from build123d import *

# Parameters (mm, degrees)
CROQUIS1_W              = 30
CROQUIS1_H              = 20
SALIENTE_EXTRUIR1_DEPTH = 24
CORTAR_EXTRUIR1_DEPTH   = 35.655446902
VACIADO1_T              = -2
CROQUIS5_W              = 16
CROQUIS5_H              = 7.775934249
CORTAR_EXTRUIR3_DEPTH   = 24
SALIENTE_EXTRUIR2_REACH = 41.699
CROQUIS6_W              = 16
CROQUIS6_H              = 3
CROQUIS7_W              = 14
CROQUIS7_H              = 14
SALIENTE_EXTRUIR3_DEPTH = 12
CROQUIS8_R              = 1.6
CORTAR_EXTRUIR5_DEPTH   = 31.528675045
CROQUIS9_R              = 2
CORTAR_EXTRUIR6_DEPTH   = 12


with BuildPart() as part:
    # Croquis1 → Saliente-Extruir1 (new body)
    with BuildSketch(Plane(origin=(0, 0, 0), x_dir=(1, 0, 0), z_dir=(0, 1, 0))):
        Rectangle(CROQUIS1_W, CROQUIS1_H)
    extrude(amount=SALIENTE_EXTRUIR1_DEPTH)

    # Croquis2 → Cortar-Extruir1 (cut, through all)
    with BuildSketch(Plane.XY.offset(10)):
        Polygon((-15, 24), (15, 3), (15, 24), align=None)
    extrude(amount=-CORTAR_EXTRUIR1_DEPTH, mode=Mode.SUBTRACT)

    # Vaciado1
    vaciado1_openings = [part.faces().sort_by_distance(p)[0] for p in [
        (0, 13.5, 0),
    ]]
    offset(amount=VACIADO1_T, openings=vaciado1_openings, kind=Kind.INTERSECTION)

    # Croquis5 → Cortar-Extruir3 (cut)
    with BuildSketch(Plane(origin=(15, 0, 0), x_dir=(0, 0, -1), z_dir=(1, 0, 0))):
        with Locations((0, 6.887967125)):
            Rectangle(CROQUIS5_W, CROQUIS5_H)
    extrude(amount=-CORTAR_EXTRUIR3_DEPTH, mode=Mode.SUBTRACT)

    # Croquis6 → Saliente-Extruir2 (add, up to next)
    with BuildSketch(Plane(origin=(15, 0, 0), x_dir=(0, 0, -1), z_dir=(1, 0, 0)), mode=Mode.PRIVATE) as saliente_extruir2_sk1:
        with Locations((0, 1.5)):
            Rectangle(CROQUIS6_W, CROQUIS6_H)
    saliente_extruir2_tool1 = extrude(saliente_extruir2_sk1.sketch, amount=-SALIENTE_EXTRUIR2_REACH, mode=Mode.PRIVATE) - part.part
    add(saliente_extruir2_tool1.solids().sort_by_distance((15, 1.5, 0))[0])

    # Croquis7 → Saliente-Extruir3 (add)
    with BuildSketch(Plane(origin=(-13, 0, 0), x_dir=(0, 0, -1), z_dir=(1, 0, 0))):
        with Locations((0, 11.74)):
            Rectangle(CROQUIS7_W, CROQUIS7_H)
    extrude(amount=SALIENTE_EXTRUIR3_DEPTH)

    # Croquis8 → Cortar-Extruir5 (cut, through all)
    with BuildSketch(Plane(origin=(-1, 0, 0), x_dir=(0, 0, -1), z_dir=(1, 0, 0))):
        with Locations((0, 11.74)):
            Circle(CROQUIS8_R)
    extrude(amount=-CORTAR_EXTRUIR5_DEPTH, mode=Mode.SUBTRACT)

    # Croquis9 → Cortar-Extruir6 (cut)
    with BuildSketch(Plane.XZ):
        with Locations(Location((7, 0, 0), (0, 0, 270))):
            Circle(CROQUIS9_R)
    extrude(amount=-CORTAR_EXTRUIR6_DEPTH, mode=Mode.SUBTRACT)


solid = part.part
CAD build for the part. Positions are in the model's coordinates, mm. A direction names the side the tool comes from. Round coordinates to 2 decimals unless told otherwise and drop trailing zeros. Order: outer loops, then holes, each group sorted by start corner. A loop starts at its lowest first (then second) coordinate and runs counter-clockwise, first axis right, second up. Notation, with made-up numbers: M -18,10.5 L 20,10.5 A13 ccw 20,24.5 Z; hole C -22.75,-11.5 d3. An arc over 180 degrees is marked long. Use one line per item in the form item = value.
Q1. Flat gauge pins, fed straight in: P1, Ø6.5, axis at x = 7, z = 0, coming from the +Y side; P2, Ø5, axis at x = -8.5, z = 5, coming from the +Y side; P3, Ø12, axis at y = 19.5, z = -5.5, coming from the +X side; P4, Ø3, axis at x = 1.5, y = 17.5, coming from the +Z side. Where does each tip first touch, or does it go through?
Recorded:
P1 = 3
P2 = 18.74
P3 = -0.78
P4 = through
Q2. Saw through at C-C on z = 0. Give the cut face in (x, y), then the cut area to 3 significant figures.
Recorded:
outline = M -15,0 L 5,0 L 5,3 L -13,3 L -13,4.74 L -1,4.74 L -1,10.14 L -15,10.14 Z; M -15,13.34 L -1,13.34 L -1,18.74 L -13,18.74 L -13,22.6 L -15,24 Z; M 9,0 L 15,0 L 15,3 L 9,3 Z
area = 242 mm^2
Q3. Saw through at A-A on x = -3. Give the cut face in (y, z), then the cut area to 3 significant figures.
Recorded:
outline = M 0,-10 L 15.6,-10 L 15.6,-8 L 3,-8 L 3,8 L 15.6,8 L 15.6,10 L 0,10 Z; M 4.74,-7 L 18.74,-7 L 18.74,7 L 4.74,7 Z; hole C 11.74,0 d3.2
area = 298 mm^2
Q4. Probe L1, parallel to Y at x = -8.5, z = 0; L2, parallel to Z at x = -9, y = 16; L3, parallel to X at y = 0.85, z = 0. List the from-to ranges inside material, lowest first.
Recorded:
L1 = 0 to 3, 4.74 to 10.14, 13.34 to 18.74
L2 = -10 to -8, -7 to 7, 8 to 10
L3 = -15 to 5, 9 to 15
Q5. Saw through at B-B on x = 7. Give the cut face in (y, z).
Recorded:
outline = M 0,-10 L 8.6,-10 L 8.6,-8 L 3,-8 L 3,-2 L 0,-2 Z; M 0,2 L 3,2 L 3,8 L 8.6,8 L 8.6,10 L 0,10 Z
Q6. Two-plate mould, pull along Y, no slides. Class faces 1 (the flat face through (-7, 18.74, 0)), 2 (the flat face through (0, 0, 0)), 3 (the flat face through (-13, 19, 2)), 4 (the flat face through (-15, 12, -2)): +Y half, -Y half, draft (parallel to the pull), parting line (faces both ways), or undercut.
Recorded:
face_1 = +Y half
face_2 = -Y half
face_3 = undercut
face_4 = draft
Q7. Saw through at D-D on y = 17. Give the cut face in (x, z).
Recorded:
outline = M -15,-10 L -5,-10 L -5,-8 L -13,-8 L -13,-7 L -1,-7 L -1,7 L -13,7 L -13,8 L -5,8 L -5,10 L -15,10 Z
Q8. Which spindle directions (+Z, -Z, +X, -X, +Y, -Y) get a long thin tool onto all of the face, cutting with end or side? Do faces 5 (the flat face through (1, 3, 0)), 6 (the flat face through (-2, 10, -8)), 7 (the flat face through (-4, 9, 10)). Say none if no direction does.
Recorded:
face_5 = +X
face_6 = +X, +Y
face_7 = +Z, +X, -X, +Y, -Y
